Solid Edge part; units mm, degrees
sketch "Sketch1" plane through (0, 0, 0) normal (0, -1, 0) x (1, 0, 0)
  line L0 (35, 25) -> (-35, 25)
  line L1 (-35, 25) -> (-35, -25)
  line L2 (-35, -25) -> (35, -25)
  line L3 (35, -25) -> (35, 25)
extrude "Protrusion1" add sketch "Sketch1" against normal blind 7
sketch "Sketch2" plane through (0, 0, 0) normal (0, -1, 0) x (1, 0, 0)
  circle A0 centre (17.5852, 0) radius 2.5
extrude "ExtrudedCutout_1" cut sketch "Sketch2" against normal blind 7
sketch "Sketch3" plane through (0, 0, 0) normal (0, -1, 0) x (1, 0, 0)
  circle A0 centre (-17.5, 0) radius 2.5
extrude "ExtrudedCutout_2" cut sketch "Sketch3" against normal blind 7
sketch "Sketch4" plane through (0, 7, 0) normal (0, 1, 0) x (-1, 0, 0)
  circle A0 centre (-29.9568, -18.7158) radius 1.5
extrude "ExtrudedCutout_3" cut sketch "Sketch4" against normal blind 7
sketch "Sketch5" plane through (0, 7, 0) normal (0, 1, 0) x (-1, 0, 0)
  circle A0 centre (30, -18.7158) radius 1.5
extrude "ExtrudedCutout_4" cut sketch "Sketch5" against normal blind 7
shell "Thinwall_2" thickness 3 removed faces 1 at (-22.6333, 7, 17.1667)
sketch "Sketch6" plane through (0, 3.5, -25) normal (0, 0, -1) x (-1, 0, 0)
  line L0 (-7.5, 1) -> (-27.5, 1)
  line L1 (-27.5, 1) -> (-27.5, -1)
  line L2 (-27.5, -1) -> (-7.5, -1)
  line L3 (-7.5, -1) -> (-7.5, 1)
extrude "ExtrudedCutout_6" cut sketch "Sketch6" against normal blind 3
sketch "Sketch7" plane through (0, 3.5, -25) normal (0, 0, -1) x (-1, 0, 0)
  line L0 (2.5, -1) -> (2.5, 1)
  line L1 (2.5, 1) -> (-2.5, 1)
  line L2 (-2.5, 1) -> (-2.5, -1)
  line L3 (-2.5, -1) -> (2.5, -1)
extrude "ExtrudedCutout_7" cut sketch "Sketch7" against normal blind 3
sketch "Sketch8" plane through (0, 3.5, -25) normal (0, 0, -1) x (-1, 0, 0)
  line L0 (27.5, 1) -> (7.5, 1)
  line L1 (7.5, 1) -> (7.5, -1)
  line L2 (7.5, -1) -> (27.5, -1)
  line L3 (27.5, -1) -> (27.5, 1)
extrude "ExtrudedCutout_8" cut sketch "Sketch8" against normal blind 3
CAD build for the part. Positions are in the model's coordinates, mm. A direction names the side the tool comes from. Coordinates: 2 decimals unless noted, no trailing zeros. Order: outer loops, then holes, each group sorted by start corner. A loop starts at its lowest first (then second) coordinate and runs counter-clockwise, first axis right, second up.
Item 1: Band-saw the part on C-C on x = -17.5. List the corners of the cut face in (y, z), plus the area to 3 significant figures.
Check sheet entries:
outline: (0, -25) - (2.5, -25) - (2.5, -22) - (3, -22) - (3, -5.5) - (7, -5.5) - (7, -2.5) - (0, -2.5) - close; (0, 2.5) - (7, 2.5) - (7, 5.5) - (3, 5.5) - (3, 22) - (7, 22) - (7, 25) - (0, 25) - close; (4.5, -25) - (7, -25) - (7, -22) - (4.5, -22) - close
area: 177 mm2
Item 2: Band-saw the part on A-A on z = 0. List the corners of the cut face in (x, y), plus the area to 3 significant figures.
Check sheet entries:
outline: (-35, 0) - (-20, 0) - (-20, 7) - (-23, 7) - (-23, 3) - (-32, 3) - (-32, 7) - (-35, 7) - close; (-15, 0) - (15.09, 0) - (15.09, 7) - (12.09, 7) - (12.09, 3) - (-12, 3) - (-12, 7) - (-15, 7) - close; (20.09, 0) - (35, 0) - (35, 7) - (32, 7) - (32, 3) - (23.09, 3) - (23.09, 7) - (20.09, 7) - close
area: 252 mm2
Item 3: 3-axis set-ups, long thin cutter, end or side, ignore diameter. For faces 1 (the face through (17, 4.5, -24)), 2 (the face through (32, 5, 3)), 3 (the face through (-20, 3, 0)): which of +Z, -Z, +X, -X, +Y, -Y reach the whole face in a straight line?
Check sheet entries:
face 1: -Z
face 2: +Y
face 3: +Y, -Y
Item 4: Drill centre lines: L1, parallel to Z at x = -30, y = 5.75; L2, parallel to Z at x = -17.5, y = 5.75; L3, parallel to X at y = 2, z = -2. Where is each one in solid material? Low to high.
Check sheet entries:
L1: z = -25 to -20.22, -17.22 to -14.22, 22 to 25
L2: z = -25 to -22, -5.5 to -2.5, 2.5 to 5.5, 22 to 25
L3: x = -35 to -19, -16 to 16.09, 19.09 to 35
Item 5: Band-saw the part on B-B on x = -30. List the corners of the cut face in (y, z), plus the area to 3 significant figures.
Check sheet entries:
outline: (0, -25) - (7, -25) - (7, -20.22) - (0, -20.22) - close; (0, -17.22) - (7, -17.22) - (7, -14.22) - (3, -14.22) - (3, 22) - (7, 22) - (7, 25) - (0, 25) - close
area: 184 mm2
Item 6: Two-plate mould, pull along Z, no slides. Class faces 4 (the face through (0, 0, 0)), 5 (the face through (-26.355, 5.028, -16.077)), 6 (the face through (0, 5, -25)): +Z half, -Z half, draft (parallel to the pull), parting line (faces both ways), or undercut.
Check sheet entries:
face 4: draft
face 5: undercut
face 6: -Z half
Item 7: Band-saw the part on D-D on z = -9. List the corners of the cut face in (x, y), plus the area to 3 significant figures.
Check sheet entries:
outline: (-35, 0) - (35, 0) - (35, 7) - (32, 7) - (32, 3) - (-32, 3) - (-32, 7) - (-35, 7) - close
area: 234 mm2
